Build history of the part. All positions in model axes, mm. Give positions to 0.01 mm unless a question says otherwise; leave off trailing zeros. Order: outer loops, then holes, each group sorted by start corner. A loop starts at its lowest first (then second) coordinate and runs counter-clockwise, first axis right, second up. Notation, with made-up numbers: M 57.25,54 L 71.25,54 A14 cw 71.25,68 Z; hole C 35,-18 d11. An arc over 180 degrees is marked long. Use CSV: the item, a comma, the result in double quotes. Start each with the question number.
Item 1: Band-saw the part on B-B on z = 5. Write the cut outline in (x, y) (3 decimals).
Item 2: Band-saw the part on A-A on x = 36. Write the cut outline in (y, z) (3 decimals).
Item 3: Pin check, flat tips, straight feed: P1, Ø10, axis at x = 13.5, y = 414, coming from the -Z side; P2, Ø3, axis at x = 29, y = 385.5, coming from the -Z side; P3, Ø1.5, axis at y = 382, z = 31, coming from the -X side; P4, Ø4, axis at x = 41.5, z = -26.5, coming from the +Y side. Stop position of each tip, or through.
Item 4: Two-plate mould, pull along Z, no slides. Class faces 1 (the cylindrical face through (21.05, 404.17, -50.05)), 2 (the cylindrical face through (-54.303, 404.079, -12.059)), 3 (the flat face through (-20.3, 457.2, 49.2)): pulls with the +Z half, pulls with the -Z half, needs draft (parallel to the pull), parting line crosses it, or undercut.
Item 5: Band-saw the part on C-C on y = 402. Write the cut outline in (x, z).
Item 6: Wall check: line 1 along Y through (x, z) = (54.75, 0) (3 decimals); line 2 along Z through (x, y) = (0, 379). Give the ranges that are in metal, low to high.
from build123d import *

# Parameters (mm, degrees)
BOSS_EXTRUDE1_START = 352.425
SKETCH1_R           = 55.626
SKETCH1_R_2         = 52.9844
BOSS_EXTRUDE1_DEPTH = 104.775
CIRPATTERN1_COUNT   = 4
CIRPATTERN2_COUNT   = 8


with BuildPart() as part:
    # Sketch1 → Boss-Extrude1 (new body)
    with BuildSketch(Plane(origin=(0, 0, 0), x_dir=(1, 0, 0), z_dir=(0, 1, 0)).offset(BOSS_EXTRUDE1_START)):
        with Locations(Location((0, 0, 0), (0, 0, 270))):
            Circle(SKETCH1_R)
        with Locations(Location((0, 0, 0), (0, 0, 270))):
            Circle(SKETCH1_R_2, mode=Mode.SUBTRACT)
    extrude(amount=BOSS_EXTRUDE1_DEPTH)

    # Sketch4 → #2 Clearance Hole1 (revolve, cut)
    with BuildSketch(Plane(origin=(0, 360.2228, 55.626), x_dir=(0, -1, 0), z_dir=(1, 0, 0))):
        Polygon((0, 0), (0, 55.596569267), (1.2192, 54.864), (1.2192, 0), align=None)
    f_2_clearance_hole1 = revolve(axis=Axis((0, 360.2228, 61.976), (0, 0, -1)), mode=Mode.SUBTRACT)

    # Sketch6 → #8 Clearance Hole1 (revolve, cut)
    with BuildSketch(Plane(origin=(21.287148609, 406.4, 51.391722875), x_dir=(0.9238795325112864, 0, -0.38268343236509056), z_dir=(0, 1, 0))):
        Polygon((0, 0), (0, 56.214674586), (2.2479, 54.864), (2.2479, 0), align=None)
    f_8_clearance_hole1 = revolve(axis=Axis((23.717188404, 406.4, 57.258357907), (-0.38268343236509056, 0, -0.9238795325112865)), mode=Mode.SUBTRACT)

    # CirPattern1: #2 Clearance Hole1 ×4 about axis
    cirpattern1_axis = Axis((0, 457.2, 0), (0, -1, 0))
    for i in range(1, CIRPATTERN1_COUNT):
        add(f_2_clearance_hole1.rotate(cirpattern1_axis, i * 360 / CIRPATTERN1_COUNT), mode=Mode.SUBTRACT)

    # CirPattern2: #8 Clearance Hole1 ×8 about axis
    cirpattern2_axis = Axis((0, 457.2, 0), (0, -1, 0))
    for i in range(1, CIRPATTERN2_COUNT):
        add(f_8_clearance_hole1.rotate(cirpattern2_axis, i * 360 / CIRPATTERN2_COUNT), mode=Mode.SUBTRACT)


solid = part.part
Model answer:
1,outline,"M -55.401,352.425 L -52.748,352.425 L -52.748,457.2 L -55.401,457.2 Z; M 52.748,352.425 L 55.401,352.425 L 55.401,457.2 L 52.748,457.2 Z"
2,outline,"M 352.425,-42.406 L 457.2,-42.406 L 457.2,-38.876 L 352.425,-38.876 Z; M 352.425,38.876 L 457.2,38.876 L 457.2,42.406 L 352.425,42.406 Z"
3,P1,"stops at z = -54.97"
3,P2,"stops at z = -48.35"
3,P3,"stops at x = -46.68"
3,P4,"passes through"
4,face 1,"undercut"
4,face 2,"parting line crosses it"
4,face 3,"needs draft"
5,outline,"C 0,0 d111.25; hole C 0,0 d105.97"
6,line 1,"y = 352.425 to 359.004, 361.442 to 457.2"
6,line 2,"z = -55.63 to -52.98, 52.98 to 55.63"
